Could you check a few things on this model? Use its own coordinates, in mm. A direction names the side the tool comes from. Give positions to 0.01 mm unless a question says otherwise; leave off trailing zeros. Loops run counter-clockwise (first coordinate to the right, second up) from the corner with the lowest first, then second, coordinate; pieces in that order, holes last. Notation, with made-up numbers: M 52.5,53.25 L 59.5,53.25 A32 cw 59.5,91.25 Z; hole C 72,-19.5 d2. An arc over 180 degrees is marked long. Use a Markdown table: item, result. Add a question column.
1) We'd pull the mould along Z, two halves only. Please class faces 3 (the cylindrical face through (-6.189, 2.613, 41.255)), 4 (the cylindrical face through (-64.805, 0.641, 89.879)), 5 (the cylindrical face through (-64.19, 3.27, 79.84)), 6 (the cylindrical face through (-0.9, 0.66, 91.14)): +Z half, -Z half, draft (parallel to the pull), parting line (faces both ways), or undercut.
2) Will these pins go through, and if not, where does the flat tip stop? pin 1 Ø1.4 at (x, z) = (-3, 3) entering from -Y; pin 2 Ø8 at (x, z) = (-7.5, 65) entering from +Y.
3) If I drill on line 1 along Z through (x, y) = (-65, 0.75); line 2 along Y through (x, z) = (-63, 36); line 3 along Z through (x, y) = (-34, 0.5), over which ranges is the centre line in solid material (lowest first)? Write a range as [from, to].
4) Suppose I cut it at C-C on y = 3.3. List the corners of the cut face in (x, z) for me.
5) Suppose I cut it at B-B on x = -31. List the corners of the cut face in (y, z) for me, and give its area (3 significant figures).
6) Which directions (+Z, -Z, +X, -X, +Y, -Y) give clear straight access to the entire face, cutting with the end or side of a thin tool? Please do faces 1 (the cylindrical face through (-6.79, 3.272, 37.917)), 2 (the cylindrical face through (-3.831, 0.641, 3.345)).
7) Suppose I cut it at A-A on z = 36. List the corners of the cut face in (x, y) for me, and give its area (3 significant figures).
Autodesk Inventor part; units mm, degrees
ref_plane "YZ Plane" through (0, 0, 0) normal (1, 0, 0) x (0, 1, 0)
ref_plane "XZ Plane" through (0, 0, 0) normal (0, 1, 0) x (-1, 0, 0)
ref_plane "XY Plane" through (0, 0, 0) normal (0, 0, 1) x (1, 0, 0)
sketch "スケッチ1" plane through (0, 0, 0) normal (0, 1, 0) x (-1, 0, 0)
  line L0 (0, 0) -> (68, 0)
  line L1 (68, 0) -> (68, 92)
  line L2 (68, 92) -> (0, 92)
  line L3 (0, 92) -> (0, 0)
  circle A0 centre (3, 89) radius 0.9
  circle A1 centre (3, 3) radius 0.9
  circle A2 centre (65, 3) radius 0.9
  circle A3 centre (65, 89) radius 0.9
  circle A4 centre (34, 60) radius 29
  circle A5 centre (61.6925, 79.7262) radius 0.9
  circle A6 centre (6.2481, 40.3574) radius 0.9
  line L4 (6.2481, 40.3574) -> (71.1751, 86.4594)
  dimension "d0" = 92
  dimension "d1" = 68
  dimension "d2" = 3
  dimension "d3" = 3
  dimension "d4" = 1.8
  dimension "d5" = 1.8
  dimension "d6" = 3
  dimension "d7" = 3
  dimension "d8" = 1.8
  dimension "d9" = 3
  dimension "d10" = 3
  dimension "d11" = 3
  dimension "d12" = 3
  dimension "d13" = 1.8
  dimension "d17" = 58
  dimension "d18" = 32
  dimension "d19" = 34
  dimension "d20" = 1.8
  dimension "d21" = 1.8
  dimension "d24" = 34
  dimension "d25" = 34
extrude "押し出し1" add sketch "スケッチ1" along normal blind 1.3
fillet "フィレット1" radius 3 4 edges at (0, 0.65, 92) (0, 0.65, 0) (-68, 0.65, 0) (-68, 0.65, 92)
sketch "スケッチ2" plane through (0, 1.3, 0) normal (0, 1, 0) x (1, 0, 0)
  circle A0 centre (-6.2481, -40.3574) radius 0.9
  circle A1 centre (-61.6925, -79.7262) radius 0.9
  circle A2 centre (-6.2481, -40.3574) radius 2.5
  circle A3 centre (-61.6925, -79.7262) radius 2.5
  point P0 (0, 0)
  dimension "d26" = 5
  dimension "d27" = 5
extrude "押し出し2" add sketch "スケッチ2" along normal blind 4
sketch "スケッチ3" plane through (0, 1.3, 0) normal (0, 1, 0) x (1, 0, 0)
  line L0 (-45.9767, -23.6507) -> (-43.3974, -22.1186)
  line L1 (-43.3974, -22.1186) -> (-39.3119, -28.9967)
  line L2 (-39.3119, -28.9967) -> (-41.8911, -30.5288)
  line L3 (-41.8911, -30.5288) -> (-45.9767, -23.6507)
  line L4 (-63, -33.7624) -> (-60.4207, -32.2303)
  line L5 (-60.4207, -32.2303) -> (-56.3352, -39.1084)
  line L6 (-56.3352, -39.1084) -> (-58.9145, -40.6405)
  line L7 (-58.9145, -40.6405) -> (-63, -33.7624)
  point P0 (0, 0)
  dimension "d31" = 8
  dimension "d32" = 8
  dimension "d33" = 3
  dimension "d34" = 3
  dimension "d35" = 0
  dimension "d46" = 22.8
extrude "押し出し3" [suppressed]
sketch "スケッチ6" plane through (0, 1.3, 0) normal (0, 1, 0) x (1, 0, 0)
  line L0 (-43.3974, -22.1186) -> (-39.3119, -28.9967)
  line L1 (-58.9145, -40.6405) -> (-63, -33.7624)
  line L2 (-58.9145, -40.6405) -> (-63, -33.7624)
  line L3 (-63, -33.7624) -> (-64.7195, -34.7838)
  line L4 (-64.7195, -34.7838) -> (-60.634, -41.6619)
  line L5 (-60.634, -41.6619) -> (-58.9145, -40.6405)
  line L6 (-39.3119, -28.9967) -> (-43.3974, -22.1186)
  line L7 (-43.3974, -22.1186) -> (-41.6779, -21.0972)
  line L8 (-41.6779, -21.0972) -> (-37.5923, -27.9753)
  line L9 (-37.5923, -27.9753) -> (-39.3119, -28.9967)
  line L10 (-64.0424, -28.8936) -> (-47.7828, -19.2356)
  line L11 (-47.7828, -19.2356) -> (-47.0244, -20.5124)
  line L12 (-47.0244, -20.5124) -> (-63.284, -30.1705)
  line L13 (-63.284, -30.1705) -> (-64.0424, -28.8936)
  point P0 (0, 0)
  dimension "d47" = 2
  dimension "d48" = 2
extrude "押し出し6" [suppressed]
sketch "スケッチ7" plane through (0, 4.8, 0) normal (0, 1, 0) x (1, 0, 0)
  line L0 (-58.9145, -40.6405) -> (-63, -33.7624)
  line L1 (-64.7195, -34.7838) -> (-60.634, -41.6619)
  line L2 (-43.3974, -22.1186) -> (-39.3119, -28.9967)
  line L3 (-39.3119, -28.9967) -> (-37.5923, -27.9753)
  line L4 (-37.5923, -27.9753) -> (-41.6779, -21.0972)
  line L5 (-41.6779, -21.0972) -> (-43.3974, -22.1186)
  line L6 (-64.7195, -34.7838) -> (-60.634, -41.6619)
  line L7 (-60.634, -41.6619) -> (-58.0547, -40.1298)
  line L8 (-58.0547, -40.1298) -> (-62.1402, -33.2517)
  line L9 (-62.1402, -33.2517) -> (-64.7195, -34.7838)
  line L10 (-41.6779, -21.0972) -> (-37.5461, -28.0532)
  line L11 (-37.5461, -28.0532) -> (-40.1254, -29.5852)
  line L12 (-40.1254, -29.5852) -> (-44.2572, -22.6293)
  line L13 (-44.2572, -22.6293) -> (-41.6779, -21.0972)
  point P0 (0, 0)
  dimension "d51" = 3
  dimension "d52" = 3
extrude "押し出し7" [suppressed]
equation "\"d3\" = d2"
equation "\"d5\" = d4"
equation "\"d6\" = d3"
equation "\"d7\" = d3"
equation "\"d8\" = d4"
equation "\"d9\" = d2"
equation "\"d10\" = d2"
equation "\"d11\" = d2"
equation "\"d12\" = d2"
equation "\"d13\" = d4"
equation "\"d19\" = 0.5 * d1"
equation "\"d21\" = d20"
equation "\"d25\" = d24"
equation "\"d27\" = d26"
equation "\"d32\" = d31"
equation "\"d34\" = d33"
equation "\"d48\" = d47"
equation "\"d52\" = d51"
properties part number "raspi-holder-top"
Answer block:
| question | item | result |
|---|---|---|
| 1 | face 3 | undercut |
| 1 | face 4 | undercut |
| 1 | face 5 | parting line |
| 1 | face 6 | +Z half |
| 2 | pin 1 | passes through |
| 2 | pin 2 | stops at y = 1.3 |
| 3 | line 1 | z = [0, 2.1], [3.9, 88.1], [89.9, 92] |
| 3 | line 2 | y = [0, 1.3] |
| 3 | line 3 | z = [0, 31], [89, 92] |
| 4 | outline | C -61.69,79.73 d5; C -6.25,40.36 d5; hole C -61.69,79.73 d1.8; hole C -6.25,40.36 d1.8 |
| 5 | outline | M 0,0 L 1.3,0 L 1.3,31.16 L 0,31.16 Z; M 0,88.84 L 1.3,88.84 L 1.3,92 L 0,92 Z |
| 5 | area | 44.6 mm^2 |
| 6 | face 1 | +Y |
| 6 | face 2 | +Y, -Y |
| 7 | outline | M -68,0 L -50.28,0 L -50.28,1.3 L -68,1.3 Z; M -17.72,0 L 0,0 L 0,1.3 L -17.72,1.3 Z |
| 7 | area | 46.1 mm^2 |
